The model under review builds one solid part; all positions refer to its coordinate system, in mm. A direction names the side the tool comes from. Coordinates: 2 decimals unless noted, no trailing zeros. Order: outer loops, then holes, each group sorted by start corner. A loop starts at its lowest first (then second) coordinate and runs counter-clockwise, first axis right, second up. Notation, with made-up numbers: (-17.75, -26) - (-10.75, -26) arc R24 cw to (-10.75, -8) - close; hole circle Ø3 at (-20, -11.5). An arc over 180 degrees is marked (long way). Answer in a Markdown table with one row per item.
Autodesk Inventor part; units mm, degrees
ref_plane "Work Plane1" through (29, 0, 0) normal (0, -1, 0) x (1, 0, 0)
ref_plane "YZ Plane" through (0, 0, 0) normal (1, 0, 0) x (0, 1, 0)
ref_plane "XZ Plane" through (0, 0, 0) normal (0, 1, 0) x (-1, 0, 0)
sketch "Sketch1" plane through (0, 0, 0) normal (0, 0, 1) x (1, 0, 0)
  line L0 (-0.0833, 0) -> (6, 0)
  line L1 (6, 0) -> (6, 1)
  line L2 (6, 1) -> (3, 1)
  line L3 (3, 1) -> (2.6932, 1)
  line L4 (2.6932, 1) -> (0, 1)
  line L5 (0, 1) -> (0, 1.75)
  line L6 (0, 1.75) -> (-1.2, 1.75)
  line L7 (-1.2, 1.75) -> (-1.2, 0.7217)
  line L8 (-1.2, 0.7217) -> (-0.5, 0.7217)
  line L9 (-0.5, 0.7217) -> (-0.0833, 0)
  line L10 (-2.64, 0) -> (7.44, 0)
  line L11 (0, -0.35) -> (0, 2.1)
  line L12 (3, 1) -> (0, 1) construction
  dimension "d1" = 3
  dimension "d2" = 0.3068
  dimension "d3" = 1.2
  dimension "d4" = 0.7
  dimension "d5" = 60
  dimension "d6" = 2
  dimension "d7" = 2
  dimension "d8" = 1.4434
  dimension "d9" = 3.5
  dimension "d26" = 6
revolve "Body" add sketch "Sketch1" angle 360 about axis through (-0.0833, 0, 0) along (1, 0, 0)
sketch "Sketch2" plane through (-1.2, 0, 0) normal (-1, 0, 0) x (0, 0, 1)
  circle A0 centre (0, 0) radius 0.7217
  line L0 (0, -2.45) -> (0, 2.45)
  line L1 (-2.45, 0) -> (2.45, 0)
  line L2 (0.7217, 0) -> (0.3608, -0.625)
  line L3 (0.3608, -0.625) -> (-0.3608, -0.625)
  line L4 (-0.3608, -0.625) -> (-0.7217, 0)
  line L5 (-0.7217, 0) -> (-0.3608, 0.625)
  line L6 (-0.3608, 0.625) -> (0.3608, 0.625)
  line L7 (0.3608, 0.625) -> (0.7217, 0)
extrude "Slot" add sketch "Sketch2" against normal up to next contours L7 A0 | A0 L2 | L6 L0 A0 | A0 L0 L3 | L0 L6 A0 | A0 L3 L0 | L4 A0 | A0 L5
fillet "Fillet1" radius 0.8 1 edges at (-1.2, -1.75, 0)
chamfer "Chamfer1" distance 0.3067 distance2 0.3067 1 edges at (6, -1, 0) measured on face at (6, 0.1182, 0.3117)
ref_plane "Work Plane1" through (29, 0, 0) normal (0, -1, 0) x (1, 0, 0)
fillet "Fillet2" radius 0.1 1 edges at (0, -1, 0)
thread "Thread2"
equation "\"d15\" = -0.5 * SPD + 0.5 * GD"
equation "\"d16\" = GUL"
equation "\"GD\" = NND"
equation "\"NLG\" = 6"
equation "\"GEL\" = 4.5"
equation "\"KOD\" = 5.7"
equation "\"KOH\" = 1.65"
equation "\"INTI\" = 1.04"
equation "\"GAL\" = 0.61345 * PTC"
equation "\"GUL\" = 0.61345 * PTC"
equation "\"BDM\" = NND"
equation "\"SW\" = 2"
equation "\"RR\" = 1.45"
equation "\"SPD\" = NND - 1.2269 * PTC"
equation "\"R\" = 0.3"
equation "\"TOA\" = 30deg"
equation "\"GD1\" = THREADDIA - 1.2269 * PTC"
equation "\"THREADDIA\" = 3"
equation "\"PTC\" = 0.5"
equation "\"NND\" = 3"
equation "\"KOH1\" = 0.2"
equation "\"E0\" = 2.303"
properties part number "M2x6 Bolt" material "Stainless Steel"
Item 1: To check wall thickness, follow line 1 (Z direction, x = 1, y = 0); line 2 (Y direction, x = 3.75, z = -0.85); line 3 (Y direction, x = 2, z = -0.8). State the ranges of each line that lie inside material, in increasing order. Write a range as from..to.
Check values:
| item | result |
|---|---|
| line 1 | -1..1 |
| line 2 | -0.53..0.53 |
| line 3 | -0.6..0.6 |
Item 2: Tool access review of faces 1 (the face through (3, 0, 1)), 2 (the face through (-0.203, 1.617, 0.67)): name each direction out of +Z, -Z, +X, -X, +Y, -Y from which nothing blocks a thin tool from reaching the whole face with its end or side.
Check values:
| item | result |
|---|---|
| face 1 | +X |
| face 2 | +X, -X |
Item 3: Clearance check with flat-ended pins moving along their axes: pin 1 Ø1.5 at (x, z) = (4.5, -1) entering from -Y; pin 2 Ø1 at (x, y) = (3, -0.5) entering from -Z. State where each tip first meets the part, or that it passes through.
Check values:
| item | result |
|---|---|
| pin 1 | y = -0.97 |
| pin 2 | z = -1 |
Item 4: We need section A-A, the plane x = 3. Write out the cut boundary in (y, z).
Check values:
| item | result |
|---|---|
| outline | circle Ø2 at (0, 0) |
